Geometry: see drawing. Coordinates: mm, zero at the bounding-box minimum. Round coordinates to 2 decimals unless told otherwise and drop trailing zeros. Loops run counter-clockwise (first coordinate to the right, second up) from the corner with the lowest first, then second, coordinate; pieces in that order, holes last.
(1) Cut plane B-B, the plane y = 270.5. Output: boundary loops of the cut face in (x, z), and give its area (3 significant figures).
(2) Cut plane C-C, the plane x = 39.5. Output: boundary loops of the cut face in (y, z) (1 decimal).
(3) Draft query along Y for the marked faces 1 and 2. Return one class per face: released by +Y, released by -Y, zero draft, split by the parting line, or undercut.
(4) Cut plane D-D, the plane z = 140. Output: boundary loops of the cut face in (x, y).
(5) Cut plane A-A, the plane x = 56. Output: boundary loops of the cut face in (y, z) (1 decimal), and give its area (3 significant figures).
(6) Line query: line 1 (Y direction, x = 20.5, z = 116) (1 decimal); line 2 (Y direction, x = 44, z = 134) (1 decimal); line 3 (Z direction, x = 31, y = 80.5). Output: solid intervals per line, ascending.
(7) First-contact query: pin 1 Ø12 at (x, y) = (24.5, 4) entering from -Z; pin 2 Ø24 at (x, z) = (40, 115) entering from +Y (1 decimal); pin 3 Ø7 at (x, y) = (37, 110.5) entering from -Z; pin 4 Ø3.5 at (x, z) = (27, 130.5) entering from -Y. Flat tips, straight axial feed; report the tip coordinate or a pass-through.
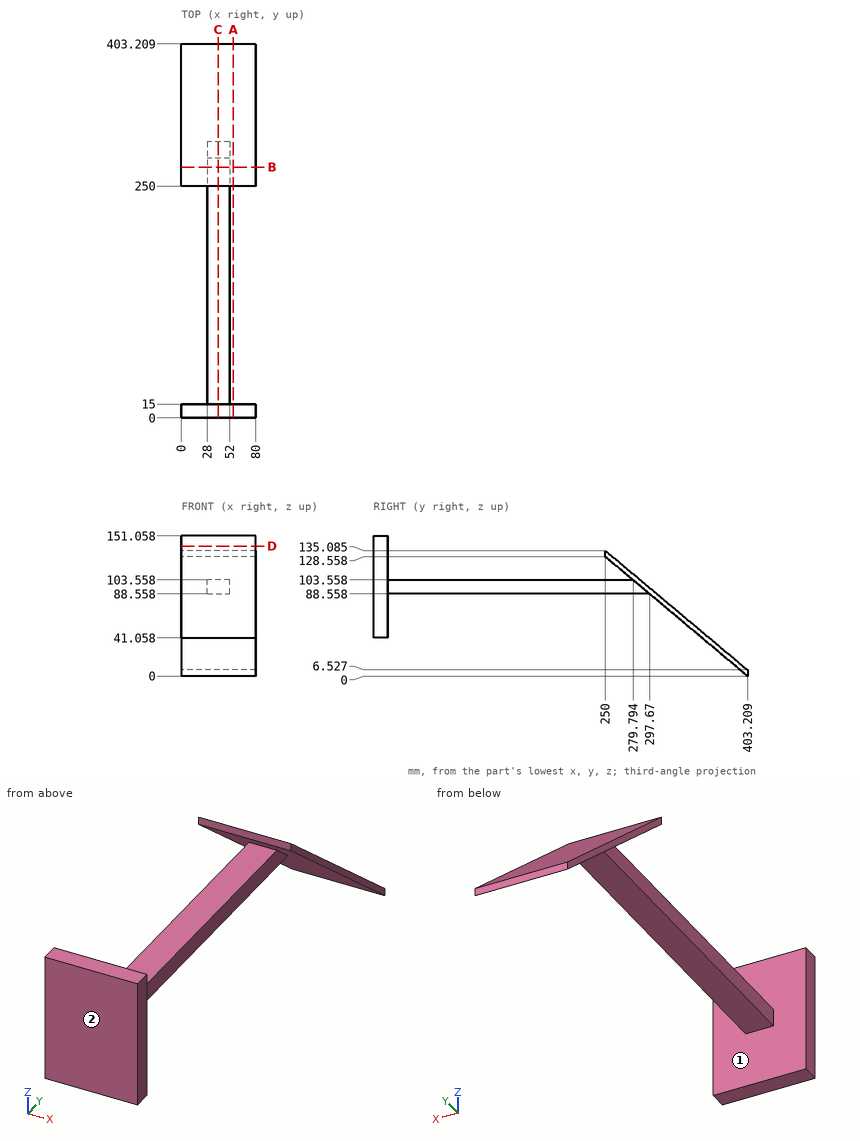
Reported:
1. outline: (0, 111.36) - (80, 111.36) - (80, 117.88) - (0, 117.88) - close; (28, 88.56) - (52, 88.56) - (52, 103.56) - (28, 103.56) - close
1. area: 882 mm2
2. outline: (0, 41.1) - (15, 41.1) - (15, 88.6) - (297.7, 88.6) - (403.2, 0) - (403.2, 6.5) - (250, 135.1) - (250, 128.6) - (279.8, 103.6) - (15, 103.6) - (15, 151.1) - (0, 151.1) - close
3. face 1: undercut
3. face 2: released by -Y
4. outline: (0, 0) - (80, 0) - (80, 15) - (0, 15) - close
5. outline: (0, 41.1) - (15, 41.1) - (15, 151.1) - (0, 151.1) - close; (250, 128.6) - (403.2, 0) - (403.2, 6.5) - (250, 135.1) - close
5. area: 2,650 mm2
6. line 1: y = 0 to 15, 265 to 272.7
6. line 2: y = 0 to 15, 250 to 251.3
6. line 3: z = 88.56 to 103.56
7. pin 1: stops at z = 41.06
7. pin 2: stops at y = 288.2
7. pin 3: stops at z = 88.56
7. pin 4: stops at y = 0
